Autodesk Inventor part; units mm, degrees
ref_plane "YZ Plane" through (0, 0, 0) normal (1, 0, 0) x (0, 1, 0)
ref_plane "XZ Plane" through (0, 0, 0) normal (0, 1, 0) x (-1, 0, 0)
ref_plane "XY Plane" through (0, 0, 0) normal (0, 0, 1) x (1, 0, 0)
sketch "Sketch1" plane through (0, 0, 0) normal (0, 1, 0) x (-1, 0, 0)
  circle A0 centre (0, 0) radius 9.15
  circle A1 centre (0, 0) radius 7.45
  dimension "d0" = 18.3
  dimension "d4" = 1.7
extrude "Extrusion2" add sketch "Sketch1" along normal blind 20
sketch "Sketch2" plane through (0, 20, 0) normal (0, 1, 0) x (1, 0, 0)
  circle A0 centre (0, 0) radius 14
  circle A1 centre (0, 0) radius 4.5
  dimension "d7" = 28
  dimension "d12" = 9
extrude "Extrusion3" add sketch "Sketch2" along normal blind 2 contours A0 | A1
thread "Thread1"
sketch "Sketch3" plane through (0, 22, 0) normal (0, 1, 0) x (1, 0, 0)
  circle A0 centre (0, 0) radius 4.5
  dimension "d13" = 9
extrude "Extrusion4" cut sketch "Sketch3" against normal through all
properties part number "Tapa"
Geometry check sheet. Reference: the model listing, model coordinates, mm. A direction names the side the tool comes from. Coordinates: 2 decimals unless noted, no trailing zeros. Order: outer loops, then holes, each group sorted by start corner. A loop starts at its lowest first (then second) coordinate and runs counter-clockwise, first axis right, second up.
Item 1: Section check D-D (z = -8.25). Enter the section's corners in (x, y), plus the area to 3 significant figures.
Item 2: Scan lines: line 1 along X through (y, z) = (21.25, 0); line 2 along Z through (x, y) = (0, 5.75). Record each from-to range of solid material in increasing order.
Item 3: Tool access check on faces 4 (the cylindrical face through (-4.919, 9.86, -7.715)), 5 (the cylindrical face through (-0.59, 21.01, -4.46)). Record the directions out of +Z, -Z, +X, -X, +Y, -Y that give a thin tool (end or side, any length) a straight path to the whole face; none if there is none.
Item 4: Mould release check, pull along X, two halves, no side actions. Record for faces 1 (the flat face through (0, 20, 5)), 2 (the cylindrical face through (12.932, 20.986, -5.362)), 3 (the flat face through (3, 0, -7)): released by +X, released by -X, zero draft, split by the parting line, or undercut.
Item 5: Depth check by flat-ended pin: pin 1 (8 mm diameter, centred on x = 2.5, y = 10.5, fed in from +Z); pin 2 (12 mm diameter, centred on y = 7, z = 7, fed in from -X); pin 3 (8 mm diameter, centred on x = 9.5, z = -9.5, fed in from -Y). Enter the tip coordinate at first touch or a pass-through.
Item 6: Section check C-C (y = 9.5). Enter the section's corners in (x, z).
Item 7: Section check A-A (z = 0). Enter the section's corners in (x, y), plus the area to 3 significant figures.
Item 8: Section check B-B (x = 0). Enter the section's corners in (y, z), plus the area to 3 significant figures.
Check sheet entries:
1. outline: (-11.31, 20) - (-3.96, 20) - (-3.96, 0) - (3.96, 0) - (3.96, 20) - (11.31, 20) - (11.31, 22) - (-11.31, 22) - close
1. area: 204 mm2
2. line 1: x = -14 to -4.5, 4.5 to 14
2. line 2: z = -9.15 to -7.45, 7.45 to 9.15
3. face 4: -Y
3. face 5: +Y, -Y
4. face 1: undercut
4. face 2: split by the parting line
4. face 3: zero draft
5. pin 1: stops at z = 9.15
5. pin 2: stops at x = -9.1
5. pin 3: stops at y = 20
6. outline: circle Ø18.3 at (0, 0); hole circle Ø14.9 at (0, 0)
7. outline: (-14, 20) - (-9.15, 20) - (-9.15, 0) - (-7.45, 0) - (-7.45, 20) - (-4.5, 20) - (-4.5, 22) - (-14, 22) - close; (4.5, 20) - (7.45, 20) - (7.45, 0) - (9.15, 0) - (9.15, 20) - (14, 20) - (14, 22) - (4.5, 22) - close
7. area: 106 mm2
8. outline: (0, -9.15) - (20, -9.15) - (20, -14) - (22, -14) - (22, -4.5) - (20, -4.5) - (20, -7.45) - (0, -7.45) - close; (0, 7.45) - (20, 7.45) - (20, 4.5) - (22, 4.5) - (22, 14) - (20, 14) - (20, 9.15) - (0, 9.15) - close
8. area: 106 mm2
